Geometry check sheet. Reference: drawing and pictorial views, mm from the part's lowest x, y, z. Give positions to 0.01 mm unless a question says otherwise; leave off trailing zeros. Write each loop counter-clockwise with the first axis right and the second up, starting at its lowest first coordinate (ties: lowest second). Pieces come first, ordered by that corner, then holes. Notation, with made-up numbers: (-36, -36) -> (-3, -36) arc R15 ccw to (-3, -30) -> close; hole circle Ø6 at (4.25, -28.75). An arc over 180 degrees is marked (long way). Write each question's results on one line, items separated by ' | '. Start each with the question number.
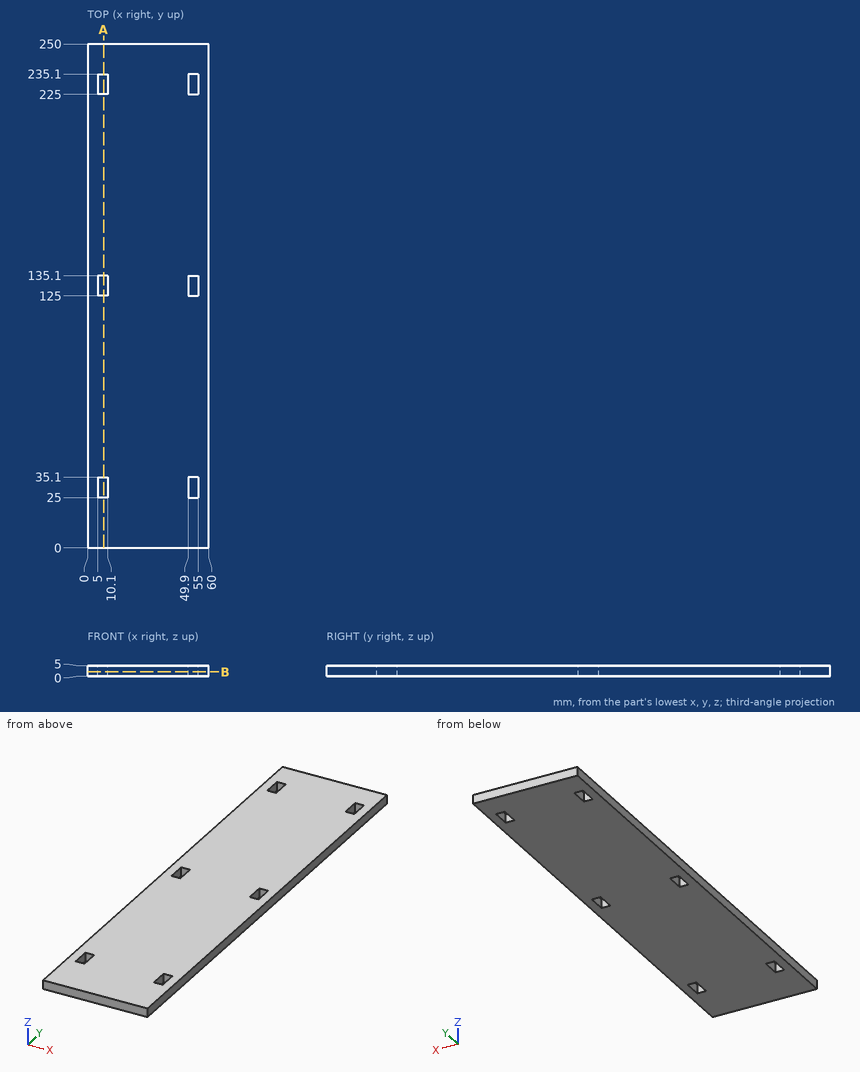
Item 1: Section check A-A on x = 8. Record the boundary of the cut face in (y, z), then the cut area to 3 significant figures.
Item 2: Thickness scan on probe 1 along Y at (x, z) = (51, 2.3); probe 2 along X at (y, z) = (226, 0.9). Record the ranges inside material, lowest first. Write a range as from..to.
Item 3: Section check B-B on z = 2. Record the boundary of the cut face in (x, y).
Check sheet entries:
1) outline: (0, 0) -> (25, 0) -> (25, 5) -> (0, 5) -> close; (35.1, 0) -> (125, 0) -> (125, 5) -> (35.1, 5) -> close; (135.1, 0) -> (225, 0) -> (225, 5) -> (135.1, 5) -> close; (235.1, 0) -> (250, 0) -> (250, 5) -> (235.1, 5) -> close | area: 1,100 mm^2
2) probe 1: y = 0..25, 35.1..125, 135.1..225, 235.1..250 | probe 2: x = 0..5, 10.1..49.9, 55..60
3) outline: (0, 0) -> (60, 0) -> (60, 250) -> (0, 250) -> close; hole (5, 25) -> (10.1, 25) -> (10.1, 35.1) -> (5, 35.1) -> close; hole (5, 125) -> (10.1, 125) -> (10.1, 135.1) -> (5, 135.1) -> close; hole (5, 225) -> (10.1, 225) -> (10.1, 235.1) -> (5, 235.1) -> close; hole (49.9, 25) -> (55, 25) -> (55, 35.1) -> (49.9, 35.1) -> close; hole (49.9, 125) -> (55, 125) -> (55, 135.1) -> (49.9, 135.1) -> close; hole (49.9, 225) -> (55, 225) -> (55, 235.1) -> (49.9, 235.1) -> close
